Autodesk Inventor part; units mm, degrees
ref_plane "YZ Plane" through (0, 0, 0) normal (1, 0, 0) x (0, 1, 0)
ref_plane "XZ Plane" through (0, 0, 0) normal (0, 1, 0) x (-1, 0, 0)
ref_plane "XY Plane" through (0, 0, 0) normal (0, 0, 1) x (1, 0, 0)
sketch "Sketch1" plane through (0, 0, 0) normal (0, 1, 0) x (-1, 0, 0)
  line L0 (-2, 0) -> (-54, 0)
  line L1 (-56, -2) -> (-56, -70)
  line L2 (-54, -72) -> (-2, -72)
  line L3 (0, -70) -> (0, -2)
  arc A0 (-2, -72) -> (0, -70) centre (-2, -70) ccw
  arc A1 (-56, -70) -> (-54, -72) centre (-54, -70) ccw
  arc A2 (-54, 0) -> (-56, -2) centre (-54, -2) ccw
  arc A3 (0, -2) -> (-2, 0) centre (-2, -2) ccw
  circle A4 centre (-4, -68) radius 2.05
  circle A5 centre (-12, -68) radius 2.05
  circle A6 centre (-20, -68) radius 2.05
  circle A7 centre (-28, -68) radius 2.05
  circle A8 centre (-36, -68) radius 2.05
  circle A9 centre (-44, -68) radius 2.05
  circle A10 centre (-52, -68) radius 2.05
  circle A11 centre (-4, -60) radius 2.05
  circle A12 centre (-12, -60) radius 2.05
  circle A13 centre (-20, -60) radius 2.05
  circle A14 centre (-28, -60) radius 2.05
  circle A15 centre (-36, -60) radius 2.05
  circle A16 centre (-44, -60) radius 2.05
  circle A17 centre (-52, -60) radius 2.05
  circle A18 centre (-4, -52) radius 2.05
  circle A19 centre (-12, -52) radius 2.05
  circle A20 centre (-20, -52) radius 2.05
  circle A21 centre (-28, -52) radius 2.05
  circle A22 centre (-36, -52) radius 2.05
  circle A23 centre (-44, -52) radius 2.05
  circle A24 centre (-52, -52) radius 2.05
  circle A25 centre (-4, -44) radius 2.05
  circle A26 centre (-12, -44) radius 2.05
  circle A27 centre (-20, -44) radius 2.05
  circle A28 centre (-28, -44) radius 2.05
  circle A29 centre (-36, -44) radius 2.05
  circle A30 centre (-44, -44) radius 2.05
  circle A31 centre (-52, -44) radius 2.05
  circle A32 centre (-4, -36) radius 2.05
  circle A33 centre (-12, -36) radius 2.05
  circle A34 centre (-20, -36) radius 2.05
  circle A35 centre (-28, -36) radius 2.05
  circle A36 centre (-36, -36) radius 2.05
  circle A37 centre (-44, -36) radius 2.05
  circle A38 centre (-52, -36) radius 2.05
  circle A39 centre (-4, -28) radius 2.05
  circle A40 centre (-12, -28) radius 2.05
  circle A41 centre (-20, -28) radius 2.05
  circle A42 centre (-28, -28) radius 2.05
  circle A43 centre (-36, -28) radius 2.05
  circle A44 centre (-44, -28) radius 2.05
  circle A45 centre (-52, -28) radius 2.05
  circle A46 centre (-4, -20) radius 2.05
  circle A47 centre (-12, -20) radius 2.05
  circle A48 centre (-20, -20) radius 2.05
  circle A49 centre (-28, -20) radius 2.05
  circle A50 centre (-36, -20) radius 2.05
  circle A51 centre (-44, -20) radius 2.05
  circle A52 centre (-52, -20) radius 2.05
  circle A53 centre (-4, -12) radius 2.05
  circle A54 centre (-12, -12) radius 2.05
  circle A55 centre (-20, -12) radius 2.05
  circle A56 centre (-28, -12) radius 2.05
  circle A57 centre (-36, -12) radius 2.05
  circle A58 centre (-44, -12) radius 2.05
  circle A59 centre (-52, -12) radius 2.05
  circle A60 centre (-4, -4) radius 2.05
  circle A61 centre (-12, -4) radius 2.05
  circle A62 centre (-20, -4) radius 2.05
  circle A63 centre (-28, -4) radius 2.05
  circle A64 centre (-36, -4) radius 2.05
  circle A65 centre (-44, -4) radius 2.05
  circle A66 centre (-52, -4) radius 2.05
  circle A67 centre (-44, -12) radius 4
  circle A68 centre (-12, -12) radius 4
  circle A69 centre (-28, -12) radius 4
  circle A70 centre (-28, -36) radius 4
  circle A71 centre (-44, -28) radius 4
  circle A72 centre (-12, -28) radius 4
  circle A73 centre (-12, -44) radius 4
  circle A74 centre (-44, -44) radius 4
  circle A75 centre (-44, -60) radius 4
  circle A76 centre (-28, -60) radius 4
  circle A77 centre (-12, -60) radius 4
  point P0 (0, 0)
  point P1 (-56, -72)
  point P2 (-56, 0)
  point P3 (0, -72)
  dimension "d0" = 56
  dimension "d1" = 72
  dimension "d2" = 2
  dimension "d3" = 4.1
  dimension "d5" = 4
  dimension "d8" = 8
  dimension "d11" = 8
  dimension "d14" = 8
  dimension "d15" = 8
  dimension "d16" = 8
  dimension "d17" = 8
  dimension "d18" = 8
  dimension "d19" = 8
  dimension "d20" = 8
  dimension "d21" = 8
  dimension "d22" = 8
  dimension "d23" = 8
  dimension "d24" = 8
extrude "Extrusion1" add sketch "Sketch1" along normal blind 2 contours A3 L3 A0 L2 A1 L1 A2 L0
properties part number "Plate 7x9"
Source: CAD feature listing. Evaluate the final solid. Frame: model axes, mm. Round coordinates to 2 decimals unless told otherwise and drop trailing zeros. Answer as a JSON object with one key per item and string values. Group by question number.
Q1. Section query A-A (z = -44). State how many separate pieces and enclosed holes the cut face has, plus the area to 3 significant figures.
Q2. Ray query, line 1 (Z direction, x = 41, y = 0.3); line 2 (Z direction, x = 46.5, y = 0.3); line 3 (X direction, y = 1.25, z = -25.5). Return the intervals inside material, ascending. Write a range as from..to.
Q3. Contact query for a flat-ended pin moving along its axis: P1, Ø4.5, axis at x = 28, z = -20, coming from the -Y side. Output: stop coordinate, or through.
Q4. Mould query, pull axis Z, two halves, no side actions, for faces 1 (the cylindrical face through (36.267, 0.986, -54.033)), 2 (the cylindrical face through (55.43, 0.99, -0.6)), 3 (the flat face through (28, 2, -41)). Classes: pulls with the +Z half, pulls with the -Z half, needs draft (parallel to the pull), parting line crosses it, or undercut.
Completed:
{
 "1": {"separate pieces": "8", "enclosed holes": "0", "area": "39.0 mm²"},
 "2": {"line 1": "-72..-62.65, -57.35..-46.65, -41.35..-30.65, -25.35..-14.65, -9.35..0", "line 2": "-72..-63.12, -56.88..-47.12, -40.88..-31.12, -24.88..-15.12, -8.88..0", "line 3": "0..8.88, 15.12..40.88, 47.12..56"},
 "3": {"P1": "y = 0"},
 "4": {"face 1": "undercut", "face 2": "pulls with the +Z half", "face 3": "needs draft"}
}
